Verification items for this drawing (mm, ordinates from the low corner). A direction names the side the tool comes from. Coordinates: 2 decimals unless noted, no trailing zeros. Order: outer loops, then holes, each group sorted by start corner. A loop starts at its lowest first (then second) coordinate and runs counter-clockwise, first axis right, second up. Notation, with made-up numbers: M -36,-23 L -13,-23 A24 cw -13,-13 Z; hole C -28.75,23.25 d6. An arc over 180 degrees is marked long. One line per item, written item: value. Start each with the question number.
1) Go/stop test with a flat-tipped pin: P1, Ø1.5, axis at y = 17.5, z = 160, coming from the +X side. Record where the tip stops, or that it passes through.
2) Sectioned sample at B-B, the plane y = 65. Enter the section's corners in (x, z), then the cut area to 3 significant figures.
3) Sectioned sample at C-C, the plane y = 45. Enter the section's corners in (x, z), then the cut area to 3 significant figures.
4) Sectioned sample at A-A, the plane z = 162.5. Enter the section's corners in (x, y), then the cut area to 3 significant figures.
5) Thickness scan on L1, parallel to Z at x = 125.75, y = 45; L2, parallel to X at y = 83, z = 160.5; L3, parallel to Y at x = 101, z = 160. Record the ranges inside material, lowest first. Write a range as from..to.
6) Access from +Z, -Z, +X, -X, +Y, -Y to the whole of each face (thin tool, end or side, straight path). Record for the marked faces 1 and 2.
7) Sectioned sample at D-D, the plane x = 76. Enter the section's corners in (y, z), then the cut area to 3 significant figures.
8) Draft check along X on the marked faces 3, 4 and 5. Enter one of: pulls with the +X half, pulls with the -X half, needs draft (parallel to the pull), parting line crosses it, or undercut.
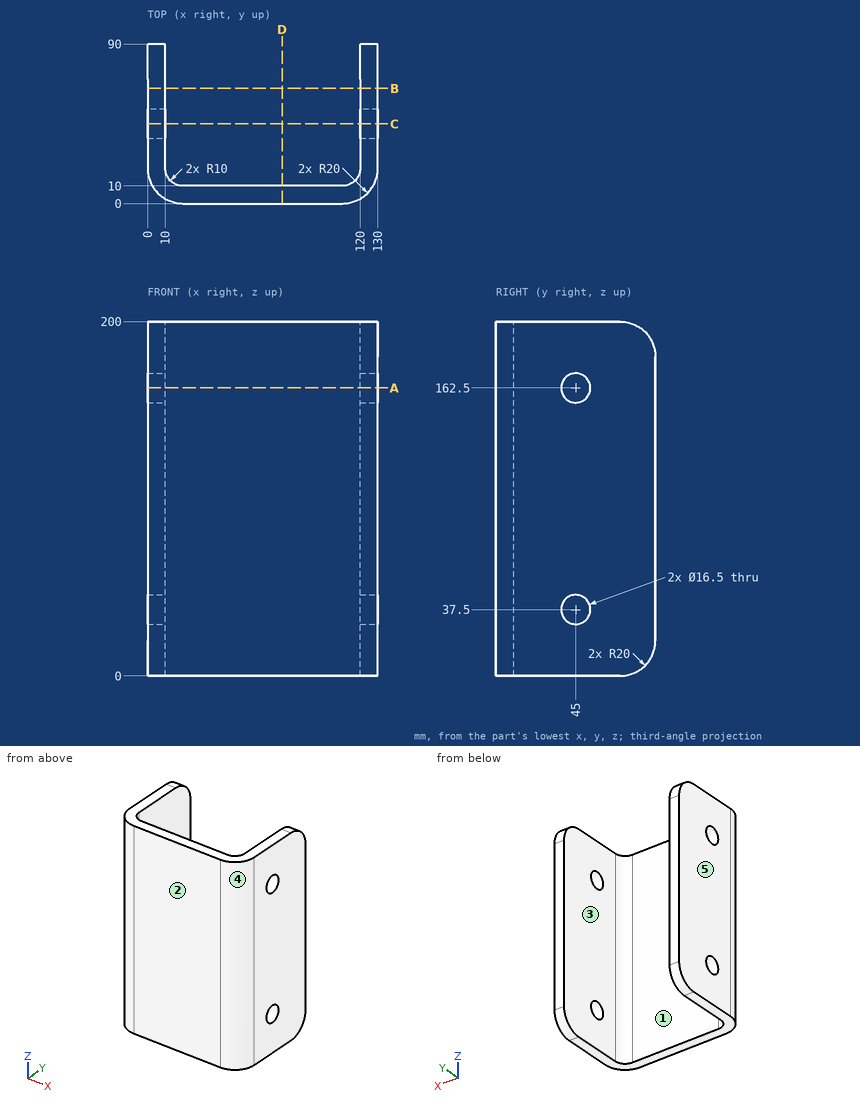
Final values:
1. P1: stops at x = 129.92
2. outline: M 0,0 L 10,0 L 10,200 L 0,200 Z; M 120,0 L 130,0 L 130,200 L 120,200 Z
2. area: 4,000 mm^2
3. outline: M 0,0 L 10,0 L 10,29.25 L 0,29.25 Z; M 0,45.75 L 10,45.75 L 10,154.25 L 0,154.25 Z; M 0,170.75 L 10,170.75 L 10,200 L 0,200 Z; M 120,0 L 130,0 L 130,29.25 L 120,29.25 Z; M 120,45.75 L 130,45.75 L 130,154.25 L 120,154.25 Z; M 120,170.75 L 130,170.75 L 130,200 L 120,200 Z
3. area: 3,340 mm^2
4. outline: M 0,20 A20 ccw 20,0 L 110,0 A20 ccw 130,20 L 130,36.75 L 120,36.75 L 120,20 A10 cw 110,10 L 20,10 A10 cw 10,20 L 10,36.75 L 0,36.75 Z; M 0,53.25 L 10,53.25 L 10,90 L 0,90 Z; M 120,53.25 L 130,53.25 L 130,90 L 120,90 Z
4. area: 2,440 mm^2
5. L1: z = 0..29.25, 45.75..154.25, 170.75..200
5. L2: x = 0..10, 120..130
5. L3: y = 0..10
6. face 1: +Z, -Z, +Y
6. face 2: +Z, -Z, +X, -X, -Y
7. outline: M 0,0 L 10,0 L 10,200 L 0,200 Z
7. area: 2,000 mm^2
8. face 3: undercut
8. face 4: pulls with the +X half
8. face 5: pulls with the -X half
